Source: CAD feature listing. Evaluate the final solid. Frame: model axes, mm. Face numbers are marked on the shaded views. A direction names the side the tool comes from. Round coordinates to 2 decimals unless told otherwise and drop trailing zeros. Loops run counter-clockwise (first coordinate to the right, second up) from the corner with the lowest first, then second, coordinate; pieces in that order, holes last. Notation, with made-up numbers: (55, 34) -> (90, 34) arc R26 ccw to (90, 72) -> close; hole circle Ø1 at (39, 49.25). An arc over 180 degrees is marked (long way). Put each result on its own line as item: value. Start each with the question number.
1. Cut plane B-B (y = 17.5). Return the cut outline in (x, z), then the cut area to 3 significant figures.
2. Set-up query: the marked faces 4 and 5. Return all of +Z, -Z, +X, -X, +Y, -Y with unobstructed straight access to the full face (end or side cutting, diameter ignored); none if empty.
3. Material intervals for L1, parallel to X at y = 45.5, z = 0.75; L2, parallel to Y at x = 6.5, z = -7.25; L3, parallel to Z at x = 8.5, y = 46.65, sorted ascending.
4. Draft query along X for the marked faces 1, 2 and 3. Return one class per face: pulls with the +X half, pulls with the -X half, needs draft (parallel to the pull), parting line crosses it, or undercut.
5. Cut plane A-A (x = 0). Return the cut outline in (y, z).
6. Contact query for flat-ended pins moving along their axis: pin 1 (1.3 mm diameter, centred on y = 57, z = -0.5, fed in from +X); pin 2 (4 mm diameter, centred on x = -4.5, y = 12, fed in from -Z); pin 3 (1 mm diameter, centred on x = -8.5, z = 3, fed in from +Y). Output: stop coordinate, or through.
```python
from build123d import *

# Parameters (mm, degrees)
SKETCH1_R                 = 12.2
BOSS_EXTRUDE1_DEPTH       = 30.8
FILLET1_R                 = 0.5
SKETCH2_R                 = 12.5
BOSS_EXTRUDE2_DEPTH       = 19
SKETCH3_R                 = 3.5
BOSS_EXTRUDE3_DEPTH       = 2.5
SKETCH4_R                 = 2
BOSS_EXTRUDE4_DEPTH       = 9
CUT_EXTRUDE1_START        = -8
CUT_EXTRUDE1_DEPTH        = 8
FILLET2_R                 = 0.5
M3X0_5_TAPPED_HOLE1_D     = 2.5
M3X0_5_TAPPED_HOLE1_DEPTH = 5
M3X0_5_TAPPED_HOLE1_TIP   = 0.751075774
SKETCH10_W                = 2
SKETCH10_H                = 1
BOSS_EXTRUDE5_DEPTH       = 4
SKETCH11_R                = 3.25
BOSS_EXTRUDE6_DEPTH       = 2


with BuildPart() as part:
    # Sketch1 → Boss-Extrude1 (new body)
    with BuildSketch(Plane(origin=(0, 0, 0), x_dir=(1, 0, 0), z_dir=(0, 1, 0))):
        with Locations(Location((0, 0, 0), (0, 0, 90))):
            Circle(SKETCH1_R)
    extrude(amount=BOSS_EXTRUDE1_DEPTH)

    # Fillet1
    fillet1_edges = [part.edges().sort_by_distance(p)[0] for p in [
        (0, 30.8, 12.2),
    ]]
    fillet(fillet1_edges, radius=FILLET1_R)

    # Sketch2 → Boss-Extrude2 (add)
    with BuildSketch(Plane(origin=(0, 30.8, 0), x_dir=(1, 0, 0), z_dir=(0, 1, 0))):
        with Locations(Location((0, 0, 0), (0, 0, 270))):
            Circle(SKETCH2_R)
    extrude(amount=BOSS_EXTRUDE2_DEPTH)

    # Sketch3 → Boss-Extrude3 (add)
    with BuildSketch(Plane(origin=(0, 49.8, 0), x_dir=(1, 0, 0), z_dir=(0, 1, 0))):
        with Locations(Location((0, 0, 0), (0, 0, 270))):
            Circle(SKETCH3_R)
    extrude(amount=BOSS_EXTRUDE3_DEPTH)

    # Sketch4 → Boss-Extrude4 (add)
    with BuildSketch(Plane(origin=(0, 52.3, 0), x_dir=(1, 0, 0), z_dir=(0, 1, 0))):
        with Locations(Location((0, 0, 0), (0, 0, 270))):
            Circle(SKETCH4_R)
    extrude(amount=BOSS_EXTRUDE4_DEPTH)

    # Sketch5 → Cut-Extrude1 (cut)
    with BuildSketch(Plane(origin=(0, 61.3, 0), x_dir=(1, 0, 0), z_dir=(0, 1, 0)).offset(CUT_EXTRUDE1_START)):
        with BuildLine():
            Line((1.5, 1.322875656), (1.5, -1.322875656))
            ThreePointArc((1.5, -1.322875656), (2, 0), (1.5, 1.322875656))
        make_face()
    extrude(amount=CUT_EXTRUDE1_DEPTH, mode=Mode.SUBTRACT)

    # Fillet2
    fillet2_edges = [part.edges().sort_by_distance(p)[0] for p in [
        (0, 49.8, -12.5),
        (0, 30.8, -12.5),
    ]]
    fillet(fillet2_edges, radius=FILLET2_R)

    # M3x0.5 Tapped Hole1
    with Locations(Plane(origin=(0, 49.8, 0), x_dir=(1, 0, 0), z_dir=(0, 1, 0))):
        with Locations((-8.5, 0), (8.5, 0)):
            Hole(M3X0_5_TAPPED_HOLE1_D / 2, depth=M3X0_5_TAPPED_HOLE1_DEPTH)
            with Locations((0, 0, -(M3X0_5_TAPPED_HOLE1_DEPTH + M3X0_5_TAPPED_HOLE1_TIP / 2))):  # 118° drill point
                Cone(0, M3X0_5_TAPPED_HOLE1_D / 2, M3X0_5_TAPPED_HOLE1_TIP, mode=Mode.SUBTRACT)

    # Sketch10 → Boss-Extrude5 (add)
    with BuildSketch(Plane.XZ):
        with Locations((-8.5, 0)):
            Rectangle(SKETCH10_W, SKETCH10_H)
        with Locations((8.5, 0)):
            Rectangle(SKETCH10_W, SKETCH10_H)
    extrude(amount=BOSS_EXTRUDE5_DEPTH)

    # Sketch11 → Boss-Extrude6 (add)
    with BuildSketch(Plane.XZ):
        with Locations(Location((0, 0, 0), (0, 0, 90))):
            Circle(SKETCH11_R)
    extrude(amount=BOSS_EXTRUDE6_DEPTH)


solid = part.part
```
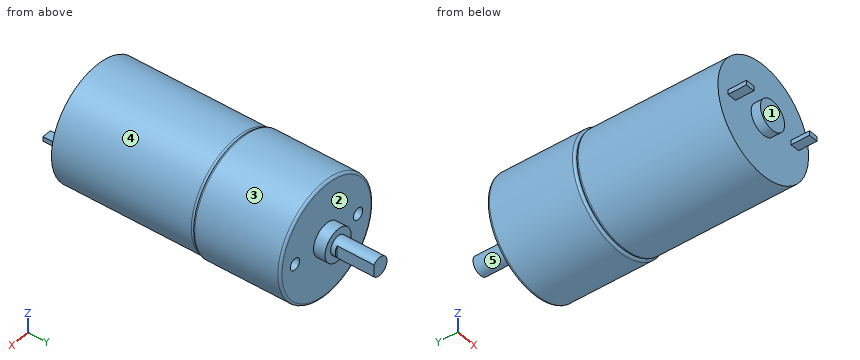
Solution:
1. outline: circle Ø24.4 at (0, 0)
1. area: 468 mm^2
2. face 4: -Y
2. face 5: +Y
3. L1: x = -12.48 to -9.5, -7.5 to 7.5, 9.5 to 12.48
3. L2: y = 0 to 49.8
3. L3: z = -9.17 to -1.25, 1.25 to 9.17
4. face 1: undercut
4. face 2: needs draft
4. face 3: parting line crosses it
5. outline: (-2, -3.25) -> (0, -3.25) -> (0, -12.2) -> (30.3, -12.2) arc R0.5 ccw to (30.8, -11.7) -> (30.8, -12) arc R0.5 ccw to (31.3, -12.5) -> (49.3, -12.5) arc R0.5 ccw to (49.8, -12) -> (49.8, -3.5) -> (52.3, -3.5) -> (52.3, -2) -> (61.3, -2) -> (61.3, 2) -> (52.3, 2) -> (52.3, 3.5) -> (49.8, 3.5) -> (49.8, 12) arc R0.5 ccw to (49.3, 12.5) -> (31.3, 12.5) arc R0.5 ccw to (30.8, 12) -> (30.8, 11.7) arc R0.5 ccw to (30.3, 12.2) -> (0, 12.2) -> (0, 3.25) -> (-2, 3.25) -> close
6. pin 1: stops at x = 1.5
6. pin 2: stops at z = -11.94
6. pin 3: stops at y = 49.8
